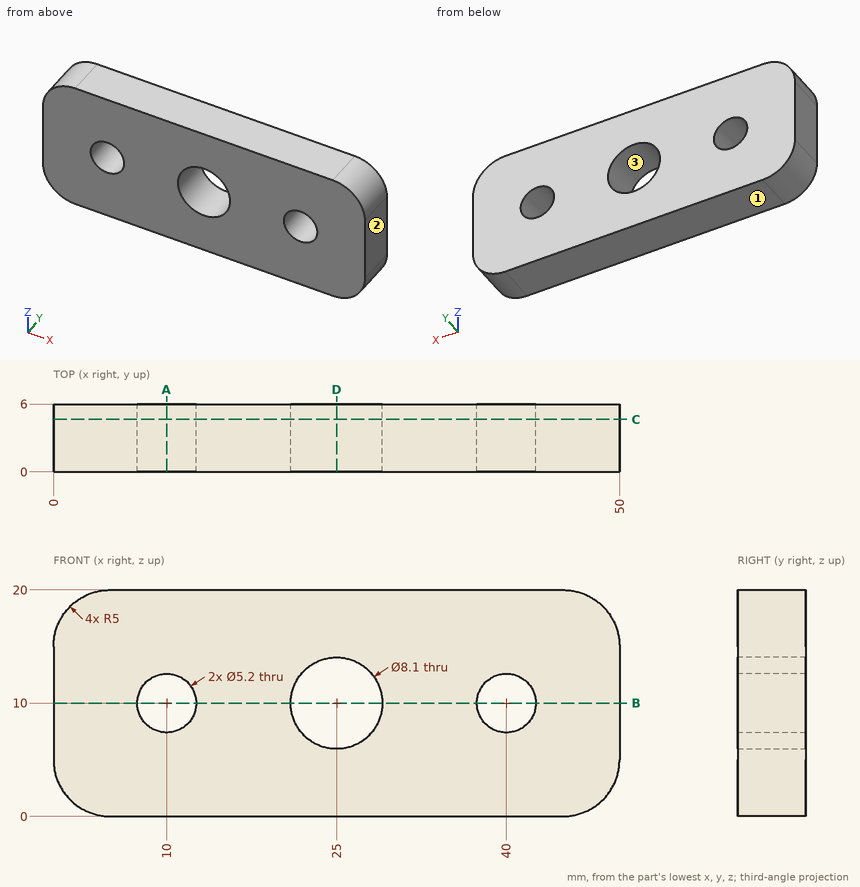
Print and shaded views of the part. All mm, measured from the part's lowest x, y and z. Coordinates: 2 decimals unless noted, no trailing zeros. Loops run counter-clockwise (first coordinate to the right, second up) from the corner with the lowest first, then second, coordinate; pieces in that order, holes last. Notation, with made-up numbers: (8.25, 2) - (50.25, 2) arc R34 cw to (50.25, 36) - close; hole circle Ø1 at (-25, -22.5). An arc over 180 degrees is marked (long way). Use one line per item in the form item = value. Start each with the question number.
1) Band-saw the part on C-C (y = 4.65). Give the cut face in (x, z), and give its area (3 significant figures).
2) Band-saw the part on B-B (z = 10). Give the cut face in (x, y).
3) Two-plate mould, pull along Z, no slides. Class the marked faces 1, 2 and 3: +Z half, -Z half, draft (parallel to the pull), parting line (faces both ways), or undercut.
4) Band-saw the part on D-D (x = 25). Give the cut face in (y, z).
5) Drill centre lines: L1, parallel to X at y = 4, z = 10; L2, parallel to Z at x = 40, y = 1.95; L3, parallel to X at y = 0.6, z = 10.75. Where is each one in solid material? Low to high. Write a range as from..to.
6) Band-saw the part on A-A (x = 10). Give the cut face in (y, z).
Check values:
q1.outline = (0, 5) arc R5 ccw to (5, 0) - (45, 0) arc R5 ccw to (50, 5) - (50, 15) arc R5 ccw to (45, 20) - (5, 20) arc R5 ccw to (0, 15) - close; hole circle Ø5.2 at (10, 10); hole circle Ø8.1 at (25, 10); hole circle Ø5.2 at (40, 10)
q1.area = 885 mm2
q2.outline = (0, 0) - (7.4, 0) - (7.4, 6) - (0, 6) - close; (12.6, 0) - (20.95, 0) - (20.95, 6) - (12.6, 6) - close; (29.05, 0) - (37.4, 0) - (37.4, 6) - (29.05, 6) - close; (42.6, 0) - (50, 0) - (50, 6) - (42.6, 6) - close
q3.face_1 = -Z half
q3.face_2 = draft
q3.face_3 = undercut
q4.outline = (0, 0) - (6, 0) - (6, 5.95) - (0, 5.95) - close; (0, 14.05) - (6, 14.05) - (6, 20) - (0, 20) - close
q5.L1 = 0..7.4, 12.6..20.95, 29.05..37.4, 42.6..50
q5.L2 = 0..7.4, 12.6..20
q5.L3 = 0..7.51, 12.49..21.02, 28.98..37.51, 42.49..50
q6.outline = (0, 0) - (6, 0) - (6, 7.4) - (0, 7.4) - close; (0, 12.6) - (6, 12.6) - (6, 20) - (0, 20) - close
